Geometry: see drawing. Coordinates: mm, zero at the bounding-box minimum. Coordinates: 2 decimals unless noted, no trailing zeros. Write each loop counter-clockwise with the first axis right and the second up, starting at its lowest first coordinate (ties: lowest second). Pieces come first, ordered by that corner, then holes. Notation, with made-up numbers: M 35,-23.75 L 90,-23.75 A11 cw 90,-9.75 Z; hole C 14,25.25 d2. An arc over 180 degrees is marked long. One line per item, written item: value. Start each with the question number.
Item 1: Ray query, L1, parallel to X at y = 20, z = 6; L2, parallel to Y at x = 284, z = 12.5; L3, parallel to X at y = 190, z = 17.25. Return the intervals inside material, ascending. Write a range as from..to.
Item 2: Cut plane C-C, the plane y = 190. Output: boundary loops of the cut face in (x, z), then the cut area to 3 significant figures.
Item 3: Cut plane D-D, the plane x = 160. Output: boundary loops of the cut face in (y, z), then the cut area to 3 significant figures.
Item 4: Cut plane B-B, the plane z = 18.75. Output: boundary loops of the cut face in (x, y), then the cut area to 3 significant figures.
Item 5: Cut plane A-A, the plane x = 285. Output: boundary loops of the cut face in (y, z), then the cut area to 3 significant figures.
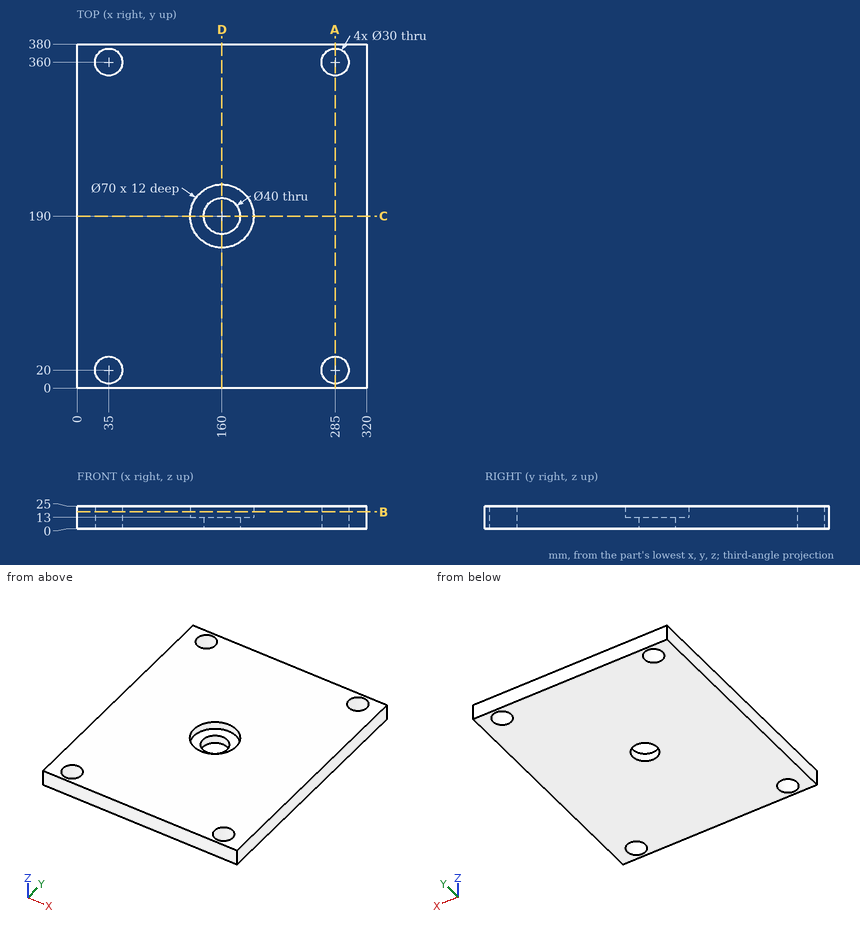
From the geometry:
1. L1: x = 0..20, 50..270, 300..320
1. L2: y = 0..5.03, 34.97..345.03, 374.97..380
1. L3: x = 0..125, 195..320
2. outline: M 0,0 L 140,0 L 140,13 L 125,13 L 125,25 L 0,25 Z; M 180,0 L 320,0 L 320,25 L 195,25 L 195,13 L 180,13 Z
2. area: 6,640 mm²
3. outline: M 0,0 L 170,0 L 170,13 L 155,13 L 155,25 L 0,25 Z; M 210,0 L 380,0 L 380,25 L 225,25 L 225,13 L 210,13 Z
3. area: 8,140 mm²
4. outline: M 0,0 L 320,0 L 320,380 L 0,380 Z; hole C 35,20 d30; hole C 35,360 d30; hole C 160,190 d70; hole C 285,20 d30; hole C 285,360 d30
4. area: 115,000 mm²
5. outline: M 0,0 L 5,0 L 5,25 L 0,25 Z; M 35,0 L 345,0 L 345,25 L 35,25 Z; M 375,0 L 380,0 L 380,25 L 375,25 Z
5. area: 8,000 mm²
